Geometry: see drawing. Coordinates: mm, zero at the bounding-box minimum. Coordinates: 2 decimals unless noted, no trailing zeros. Order: outer loops, then holes, each group sorted by start corner. A loop starts at its lowest first (then second) coordinate and runs counter-clockwise, first axis right, second up.
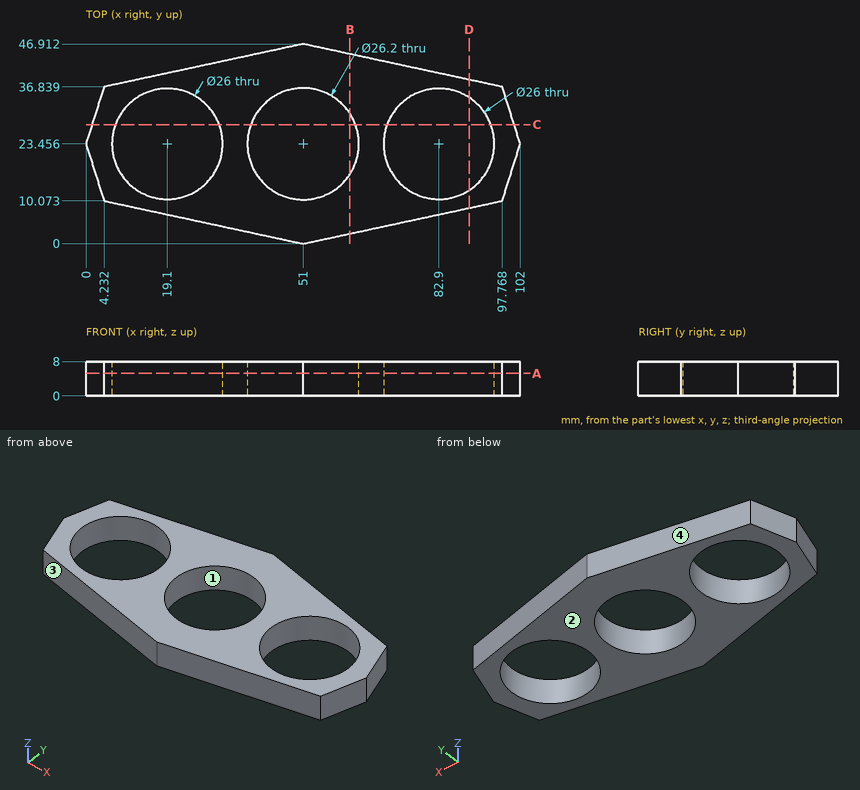
Item 1: Draft query along Y for the marked faces 1, 2, 3 and 4. Return one class per face: pulls with the +Y half, pulls with the -Y half, needs draft (parallel to the pull), parting line crosses it, or undercut.
Response values:
face 1: undercut
face 2: needs draft
face 3: pulls with the -Y half
face 4: pulls with the +Y half
Item 2: Cut plane A-A on z = 5.25. Return loops of the section in (x, y).
Response values:
outline: (0, 23.46) - (4.23, 10.07) - (51, 0) - (97.77, 10.07) - (102, 23.46) - (97.77, 36.84) - (51, 46.91) - (4.23, 36.84) - close; hole circle Ø26 at (19.1, 23.46); hole circle Ø26.2 at (51, 23.46); hole circle Ø26 at (82.9, 23.46)
Item 3: Cut plane C-C on y = 28. Return loops of the section in (x, z).
Response values:
outline: (1.44, 0) - (6.92, 0) - (6.92, 8) - (1.44, 8) - close; (31.28, 0) - (38.71, 0) - (38.71, 8) - (31.28, 8) - close; (63.29, 0) - (70.72, 0) - (70.72, 8) - (63.29, 8) - close; (95.08, 0) - (100.56, 0) - (100.56, 8) - (95.08, 8) - close
Item 4: Ray query, probe 1 along X at (y, z) = (32, 5.25); probe 2 along X at (y, z) = (27.5, 3) (1 decimal); probe 3 along Y at (x, z) = (51, 2) (1 decimal). Return the intervals inside material, ascending.
Response values:
probe 1: x = 2.7 to 9.3, 28.9 to 41.07, 60.93 to 73.1, 92.7 to 99.3
probe 2: x = 1.3 to 6.7, 31.5 to 38.5, 63.5 to 70.5, 95.3 to 100.7
probe 3: y = 0 to 10.4, 36.6 to 46.9
Item 5: Pin query (flat end, axial travel): pin 1 Ø4 at (x, z) = (32, 6.5) entering from +Y; pin 2 Ø2 at (y, z) = (14, 6) entering from +X; pin 3 Ø1 at (x, z) = (17.5, 5.5) entering from +Y (1 decimal). Return the tip coordinate at first contact, or that it passes through.
Response values:
pin 1: stops at y = 43.25
pin 2: stops at x = 99.33
pin 3: stops at y = 39.8
Item 6: Cut plane B-B on x = 62. Return loops of the section in (y, z).
Response values:
outline: (2.37, 0) - (16.34, 0) - (16.34, 8) - (2.37, 8) - close; (30.57, 0) - (44.54, 0) - (44.54, 8) - (30.57, 8) - close
Item 7: Cut plane D-D on x = 90. Return loops of the section in (y, z).
Response values:
outline: (8.4, 0) - (12.57, 0) - (12.57, 8) - (8.4, 8) - close; (34.35, 0) - (38.51, 0) - (38.51, 8) - (34.35, 8) - close
